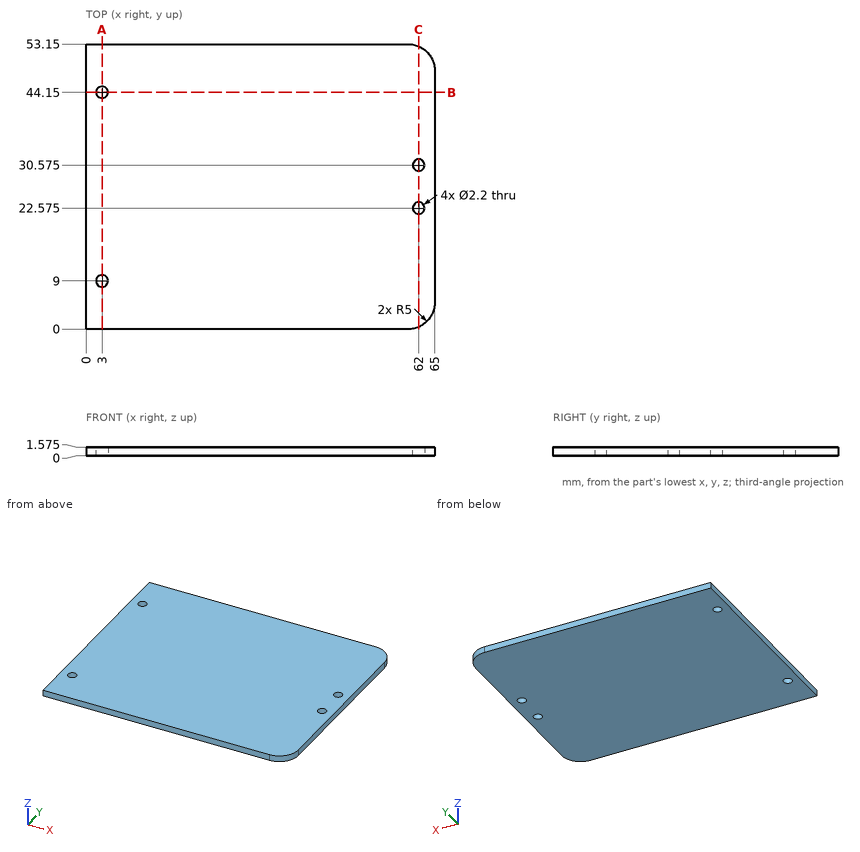
Study the drawing (mm; zero at the part's minimum x, y, z) and answer. Coordinates: 2 decimals unless noted, no trailing zeros. Write each loop counter-clockwise with the first axis right and the second up, starting at its lowest first coordinate (ties: lowest second). Pieces come first, ordered by that corner, then holes.
Q1. A cutting plane is placed at B-B, the plane y = 44.15. Give the vertices of the cut face in (x, z) (1 decimal).
Q2. Each of these flat-tipped pins is pushed along its axis until it touches: pin 1 Ø2 at (x, y) = (3, 9) entering from +Z; pin 2 Ø3 at (x, y) = (3, 44.15) entering from -Z. Where does it stop, or does it pass through?
Q3. A cutting plane is placed at A-A, the plane x = 3. State how many separate pieces and enclosed holes the cut face has.
Q4. A cutting plane is placed at C-C, the plane x = 62. Give the vertices of the cut face in (y, z) (1 decimal).
Q5. Find the intervals of material crossed by line 1 (Y direction, x = 3, z = 1.2); line 2 (Y direction, x = 62, z = 1.15) (1 decimal); line 3 (X direction, y = 45, z = 0.5), in increasing order.
Findings below:
1. outline: (0, 0) - (1.9, 0) - (1.9, 1.6) - (0, 1.6) - close; (4.1, 0) - (65, 0) - (65, 1.6) - (4.1, 1.6) - close
2. pin 1: passes through
2. pin 2: stops at z = 0
3. separate pieces: 3
3. enclosed holes: 0
4. outline: (0.4, 0) - (21.5, 0) - (21.5, 1.6) - (0.4, 1.6) - close; (23.7, 0) - (29.5, 0) - (29.5, 1.6) - (23.7, 1.6) - close; (31.7, 0) - (52.7, 0) - (52.7, 1.6) - (31.7, 1.6) - close
5. line 1: y = 0 to 7.9, 10.1 to 43.05, 45.25 to 53.15
5. line 2: y = 0.4 to 21.5, 23.7 to 29.5, 31.7 to 52.7
5. line 3: x = 0 to 2.3, 3.7 to 65
